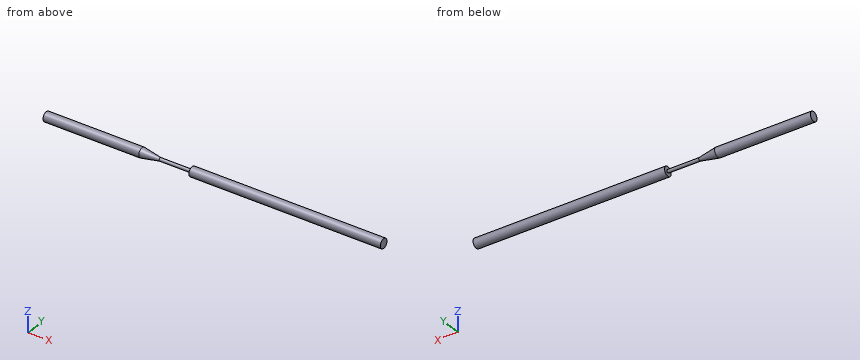
```python
from build123d import *

# Parameters (mm, degrees)
F0_R      = 6
F1_DEPTH  = 120
F1_FACE_R = 6
F3_R      = 2
F5_R      = 2
F6_DEPTH  = 40
F8_R      = 6
F9_DEPTH  = 240


with BuildPart() as f1:
    # F0 (on Right) → F1 (new body)
    with BuildSketch(Plane.YZ):
        Circle(F0_R)
    extrude(amount=F1_DEPTH)

    # F1_face (on face) → F4 section 0
    with BuildSketch(Plane.YZ.offset(120)):
        Circle(F1_FACE_R)
    # F3 (on offset) → F4 section 1
    with BuildSketch(Plane.YZ.offset(142.685)):
        Circle(F3_R)
    loft()

    # F5 (on offset) → F6 (join)
    with BuildSketch(Plane.YZ.offset(142.685)):
        Circle(F5_R)
    extrude(amount=F6_DEPTH)

    # F8 (on offset) → F9 (join)
    with BuildSketch(Plane.YZ.offset(182.685)):
        Circle(F8_R)
    extrude(amount=F9_DEPTH)


solid = f1.part
```
Source: CAD feature listing. Evaluate the final solid. Frame: model axes, mm. Give positions to 0.01 mm unless a question says otherwise; leave off trailing zeros. Loops run counter-clockwise (first coordinate to the right, second up) from the corner with the lowest first, then second, coordinate; pieces in that order, holes last. Notation, with made-up numbers: (24, 33.25) - (61, 33.25) arc R27 ccw to (61, 64.25) - close; hole circle Ø11 at (15.5, 69). An arc over 180 degrees is marked (long way). Use CSV: the item, a comma, the result in double quotes. Start each with the question number.
1. Section A-A (y = 0). Output: boundary loops of the cut face in (x, z) (3 decimals), then the cut area to 3 significant figures.
2. Ray query, L1, parallel to Y at x = 264, z = -0.25; L2, parallel to Y at x = 397, z = 1; L3, parallel to Z at x = 376.5, y = 0.75. Return the intervals inside material, ascending.
3. Pin query (flat end, axial travel): pin 1 (6 mm diameter, centred on x = 81.5, z = -4, fed in from -Y); pin 2 (1.5 mm diameter, centred on x = 92.5, z = -3.5, fed in from -Y); pin 3 (3 mm diameter, centred on y = -1, z = -0.5, fed in from -X). Return the tip coordinate at first contact, or that it passes through.
4. Section B-B (x = 168.5). Output: boundary loops of the cut face in (y, z), then the cut area to 3 significant figures.
5. Section C-C (x = 373.5). Output: boundary loops of the cut face in (y, z), then the cut area to 3 significant figures.
Response:
1,outline,"(0, -6) - (120, -6) - (142.685, -2) - (182.685, -2) - (182.685, -6) - (422.685, -6) - (422.685, 6) - (182.685, 6) - (182.685, 2) - (142.685, 2) - (120, 6) - (0, 6) - close"
1,area,"4,660 mm²"
2,L1,"-5.99 to 5.99"
2,L2,"-5.92 to 5.92"
2,L3,"-5.95 to 5.95"
3,pin 1,"y = -5.92"
3,pin 2,"y = -5.33"
3,pin 3,"x = 0"
4,outline,"circle Ø4 at (0, 0)"
4,area,"12.6 mm²"
5,outline,"circle Ø12 at (0, 0)"
5,area,"113 mm²"
